from build123d import *

# Parameters (mm, degrees)
SKIZZE1_W                       = 40
SKIZZE1_H                       = 75
AUFSATZ_LINEAR_AUSTRAGEN1_DEPTH = 6
AUFSATZ_LINEAR_AUSTRAGEN2_DEPTH = 22
SKIZZE3_W                       = 10.5
SKIZZE3_H                       = 5.5
SCHNITT_LINEAR_AUSTRAGEN1_DEPTH = 17
SKIZZE4_R                       = 3
SCHNITT_LINEAR_AUSTRAGEN2_DEPTH = 79.368616167
SKIZZE5_W                       = 40
SKIZZE5_H                       = 25
AUFSATZ_LINEAR_AUSTRAGEN3_DEPTH = 40
SKIZZE6_W                       = 29.5
SKIZZE6_H                       = 29.5
SCHNITT_LINEAR_AUSTRAGEN3_DEPTH = 20
SKIZZE7_R                       = 14.75
SCHNITT_LINEAR_AUSTRAGEN4_DEPTH = 84.066238629


with BuildPart() as part:
    # Skizze1 → Aufsatz-Linear austragen1 (new body)
    with BuildSketch(Plane.XY):
        with Locations((0, 37.5)):
            Rectangle(SKIZZE1_W, SKIZZE1_H)
    extrude(amount=AUFSATZ_LINEAR_AUSTRAGEN1_DEPTH)

    # Skizze2 → Aufsatz-Linear austragen2 (add)
    with BuildSketch(Plane(origin=(0, 75, 0), x_dir=(1, 0, 0), z_dir=(0, 1, 0))):
        Polygon((8.513843876, -6), (-8.513843876, -6), (-9.8, -10.8), (9.8, -10.8), align=None)
    extrude(amount=-AUFSATZ_LINEAR_AUSTRAGEN2_DEPTH)

    # Skizze3 → Schnitt-Linear austragen1 (cut)
    with BuildSketch(Plane(origin=(0, 75, 0), x_dir=(1, 0, 0), z_dir=(0, 1, 0))):
        with Locations((0, -5.4)):
            Rectangle(SKIZZE3_W, SKIZZE3_H)
    extrude(amount=-SCHNITT_LINEAR_AUSTRAGEN1_DEPTH, mode=Mode.SUBTRACT)

    # Skizze4 → Schnitt-Linear austragen2 (cut, through all)
    with BuildSketch(Plane.XY.offset(10.8)):
        with Locations((0, 63)):
            Circle(SKIZZE4_R)
    extrude(amount=-SCHNITT_LINEAR_AUSTRAGEN2_DEPTH, mode=Mode.SUBTRACT)

    # Skizze5 → Aufsatz-Linear austragen3 (add)
    with BuildSketch(Plane(origin=(0, 0, 0), x_dir=(-1, 0, 0), z_dir=(0, 0, -1))):
        with Locations((0, 12.5)):
            Rectangle(SKIZZE5_W, SKIZZE5_H)
    extrude(amount=AUFSATZ_LINEAR_AUSTRAGEN3_DEPTH)

    # Skizze6 → Schnitt-Linear austragen3 (cut)
    with BuildSketch(Plane(origin=(0, 25, 0), x_dir=(1, 0, 0), z_dir=(0, 1, 0))):
        with Locations((0, 22)):
            Rectangle(SKIZZE6_W, SKIZZE6_H)
    extrude(amount=-SCHNITT_LINEAR_AUSTRAGEN3_DEPTH, mode=Mode.SUBTRACT)

    # Skizze7 → Schnitt-Linear austragen4 (cut, through all)
    with BuildSketch(Plane(origin=(0, 5, 0), x_dir=(1, 0, 0), z_dir=(0, 1, 0))):
        with Locations(Location((0, 22, 0), (0, 0, 270))):
            Circle(SKIZZE7_R)
    extrude(amount=-SCHNITT_LINEAR_AUSTRAGEN4_DEPTH, mode=Mode.SUBTRACT)


solid = part.part
Can you work these out from the model? Positions are in its coordinate system, mm. A direction names the side the tool comes from. Coordinates: 2 decimals unless noted, no trailing zeros. Order: outer loops, then holes, each group sorted by start corner. A loop starts at its lowest first (then second) coordinate and runs counter-clockwise, first axis right, second up. Notation, with made-up numbers: (45, 16.5) - (63, 16.5) arc R33 ccw to (63, 55.5) - close; hole circle Ø7 at (-32.75, 60.25). An arc over 180 degrees is marked (long way). Answer as a JSON object with one key per item and string values. Group by question number.
Q1. We'd pull the mould along X, two halves only. Please class faces 6 (the face through (20, 20, -12)), 7 (the face through (-5.25, 67, 5)), 8 (the face through (0, 75, 2)): +X half, -X half, draft (parallel to the pull), parting line (faces both ways), or undercut.
Q2. Will these pins go through, and if not, where does the flat tip stop? P1, Ø22, axis at x = 4.5, y = 11.5, coming from the +Z side; P2, Ø9.5, axis at x = 0, y = 63, coming from the -Z side; P3, Ø7.5, axis at x = -9.5, z = -13.5, coming from the +Y side; P4, Ø7.5, axis at x = 6.5, z = -18, coming from the +Y side.
Q3. On a 3-axis mill with a long thin cutter (end or side, diameter ignored), from which of +Z, -Z, +X, -X, +Y, -Y can I reach the whole of each face in a straight line? I mean faces 1 (the face through (0, 50, 0)), 2 (the face through (-12, 5, -33)), 3 (the face through (9.166, 64.154, 8.434)), 4 (the face through (0, 53, 8)), 5 (the face through (0.649, 2.535, -36.736)). Say none if no direction works.
Q4. Imagine slicing it at B-B (z = -30.5). Please give me the cut outline in (x, y), and give its area (3 significant figures).
Q5. I need wall thicknesses on line 1 (Y direction, x = 0, z = 9); line 2 (X direction, y = 15, z = -16.5); line 3 (Y direction, x = 0, z = 1.35). Which ranges of each line are inside material? Lowest first, please. Write a range as from..to.
Q6. Imagine slicing it at A-A (y = 63). Please give me the cut outline in (x, z).
Q7. Imagine slicing it at D-D (y = 10). Please give me the cut outline in (x, z), and give its area (3 significant figures).
Q8. Imagine slicing it at C-C (x = 12.5). Please give me the cut outline in (y, z).
Determined:
{
 "1": {"face 6": "+X half", "face 7": "undercut", "face 8": "draft"},
 "2": {"P1": "stops at z = 6", "P2": "stops at z = 0", "P3": "stops at y = 5", "P4": "passes through"},
 "3": {"face 1": "-Z, +X, -X, +Y", "face 2": "+Y", "face 3": "+X, +Y, -Y", "face 4": "+Z, +X, -X, -Y", "face 5": "+Y, -Y"},
 "4": {"outline": "(-20, 0) - (-12.05, 0) - (-12.05, 5) - (-14.75, 5) - (-14.75, 25) - (-20, 25) - close; (12.05, 0) - (20, 0) - (20, 25) - (14.75, 25) - (14.75, 5) - (12.05, 5) - close", "area": "289 mm2"},
 "5": {"line 1": "y = 53..60, 66..75", "line 2": "x = -20..-14.75, 14.75..20", "line 3": "y = 0..60, 66..75"},
 "6": {"outline": "(-20, 0) - (-3, 0) - (-3, 2.65) - (-5.25, 2.65) - (-5.25, 8.15) - (-3, 8.15) - (-3, 10.8) - (-9.8, 10.8) - (-8.51, 6) - (-20, 6) - close; (3, 0) - (20, 0) - (20, 6) - (8.51, 6) - (9.8, 10.8) - (3, 10.8) - (3, 8.15) - (5.25, 8.15) - (5.25, 2.65) - (3, 2.65) - close"},
 "7": {"outline": "(-20, -40) - (20, -40) - (20, 6) - (-20, 6) - close; hole (-14.75, -36.75) - (14.75, -36.75) - (14.75, -7.25) - (-14.75, -7.25) - close", "area": "970 mm2"},
 "8": {"outline": "(0, -40) - (25, -40) - (25, -36.75) - (5, -36.75) - (5, -29.83) - (0, -29.83) - close; (0, -14.17) - (5, -14.17) - (5, -7.25) - (25, -7.25) - (25, 0) - (75, 0) - (75, 6) - (0, 6) - close"}
}
